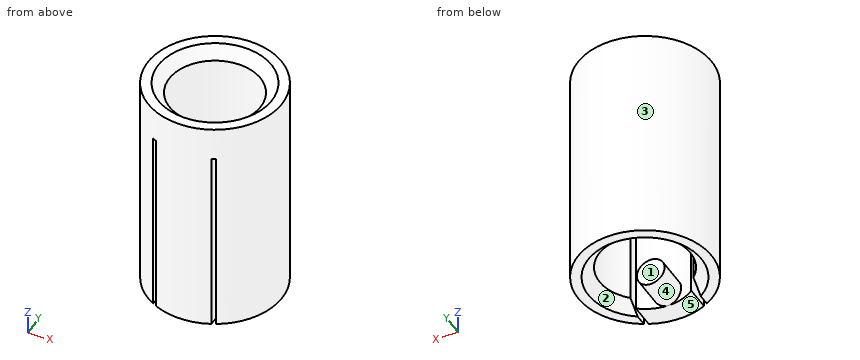
from build123d import *

# Parameters (mm, degrees)
F0_R     = 6.02
F0_R_2   = 4.1
F1_DEPTH = 20
F3_R     = 1.25
F4_DEPTH = 4
F5_W     = 0.35
F5_H     = 17
F6_DEPTH = 2.5
F7_SIZE  = 1


with BuildPart() as f1:
    # F0 (on Top) → F1 (new body)
    with BuildSketch(Plane.XY):
        Circle(F0_R)
        Circle(F0_R_2, mode=Mode.SUBTRACT)
    extrude(amount=F1_DEPTH)

    # F3 (on offset) → F4 (join)
    with BuildSketch(Plane.XZ.offset(5)):
        with Locations((0, 1.25)):
            Circle(F3_R)
    extrude(amount=-F4_DEPTH)

    # F5 (on offset) → F6 (cut, symmetric)
    with BuildSketch(Plane.XZ.offset(5)):
        with Locations((-2.675, 8.5)):
            Rectangle(F5_W, F5_H)
        with Locations((2.675, 8.5)):
            Rectangle(F5_W, F5_H)
    extrude(amount=F6_DEPTH, both=True, mode=Mode.SUBTRACT)

    # F7
    f7_edges = [f1.edges().sort_by_distance(p)[0] for p in [
        (-4.1, 0, 20),
        (-1.600781, 3.774586, 0),
    ]]
    chamfer(f7_edges, length=F7_SIZE)


solid = f1.part
Part model, mm, in its own coordinate system. Face numbers are marked on the shaded views. A direction names the side the tool comes from. Coordinates: 2 decimals unless noted, no trailing zeros. Order: outer loops, then holes, each group sorted by start corner. A loop starts at its lowest first (then second) coordinate and runs counter-clockwise, first axis right, second up.
(1) Pin check, flat tips, straight feed: pin 1 Ø2 at (x, z) = (-5, 14.5) entering from -Y; pin 2 Ø2 at (x, z) = (5, 9) entering from +Y; pin 3 Ø1.2 at (y, z) = (-4.5, 4.5) entering from -X; pin 4 Ø4 at (x, z) = (1.5, 8.5) entering from +Y. Stop position of each tip, or through.
Check sheet entries:
pin 1: stops at y = -4.5
pin 2: stops at y = 4.5
pin 3: stops at x = -4.59
pin 4: stops at y = 6.02
(2) Slice it at C-C, the plane z = 17.5. Write the cut outline in (x, y).
Check sheet entries:
outline: circle Ø12.04 at (0, 0); hole circle Ø8.2 at (0, 0)
(3) Slice it at D-D, the plane y = -1.75. State how many separate pieces and enclosed holes the cut face has, and give its area (3 significant figures).
Check sheet entries:
separate pieces: 3
enclosed holes: 0
area: 84.8 mm2
(4) Tool access for the marked faces 1 and 2: list every direction of +Z, -Z, +X, -X, +Y, -Y with a clear straight run to the whole face (end or side of a thin tool).
Check sheet entries:
face 1: +Z, -Z
face 2: -Z
(5) Slice it at A-A, the plane y = 0. Write the cut outline in (x, z).
Check sheet entries:
outline: (-6.02, 0) - (-5.1, 0) - (-4.1, 1) - (-4.1, 19) - (-5.1, 20) - (-6.02, 20) - close; (4.1, 1) - (5.1, 0) - (6.02, 0) - (6.02, 20) - (5.1, 20) - (4.1, 19) - close
(6) Slice it at B-B, the plane z = 10.5. Write the cut outline in (x, y), and give its area (3 significant figures).
Check sheet entries:
outline: (-2.85, -5.3) - (-2.85, -2.95) arc R4.1 cw (long way) to (2.85, -2.95) - (2.85, -5.3) arc R6.02 ccw (long way) to start; (-2.5, -5.48) arc R6.02 ccw to (2.5, -5.48) - (2.5, -3.25) arc R4.1 cw to (-2.5, -3.25) - close
area: 59.4 mm2
(7) Probe L1, parallel to Y at x = 0, z = 13.5; L2, parallel to X at y = -3.5, z = 8. List the from-to ranges inside material, lowest first.
Check sheet entries:
L1: y = -6.02 to -4.1, 4.1 to 6.02
L2: x = -4.9 to -2.85, -2.5 to -2.14, 2.14 to 2.5, 2.85 to 4.9
(8) Pull direction X, two halves, no side cores. Call the marked faces 3, 4 and 5: pulls with the +X half, pulls with the -X half, needs draft (parallel to the pull), parting line crosses it, or undercut.
Check sheet entries:
face 3: parting line crosses it
face 4: undercut
face 5: needs draft
